Can you work these out from the model? Positions are in its coordinate system, mm. A direction names the side the tool comes from. Round coordinates to 2 decimals unless told otherwise and drop trailing zeros. Write each loop counter-clockwise with the first axis right and the second up, starting at its lowest first coordinate (ties: lowest second). Pieces come first, ordered by that corner, then holes. Notation, with made-up numbers: M 26,-21 L 35,-21 A11 ccw 35,-17 Z; hole C 66.5,-24 d3. An arc over 180 degrees is marked long. Answer as a JSON object with one key per item and string values. Group by question number.
1) Please list where these lines run through material, in increasing order: L1, parallel to Y at x = 15.5, z = 42.75; L2, parallel to X at y = -15, z = 44. Write a range as [from, to].
2) On a 3-axis mill with a long thin cutter (end or side, diameter ignored), from which of +Z, -Z, +X, -X, +Y, -Y can I reach the whole of each face in a straight line? I mean faces 4 (the cylindrical face through (16.421, 16.345, 43.237)), 5 (the flat face through (8, 23, 4)), 6 (the flat face through (0, -20, 24)). Say none if no direction works.
3) If we mould it in two halves opening along Z, with no side actions, what happens to faces 1 (the conical face through (-15.55, 15.29, 38.18)), 2 (the flat face through (0, -21, 5)), 3 (the flat face through (20.3, 0.1, 10))? For each: +Z half, -Z half, draft (parallel to the pull), parting line (faces both ways), or undercut.
4) I'm going to push flat-ended pins straight in: pin 1 Ø11 at (x, z) = (-0.5, 42.5) entering from +Y; pin 2 Ø10 at (x, y) = (9, 1) entering from +Z; pin 3 Ø1.5 at (x, y) = (-1, -15.5) entering from +Z. Where does each tip first touch, or does it pass through?
5) Suppose I cut it at A-A, the plane z = 46. Write out the boundary of the cut face in (x, y).
6) Suppose I cut it at B-B, the plane y = 0. Write out the boundary of the cut face in (x, z).
from build123d import *

# Parameters (mm, degrees)
EXTRUDE_1_DEPTH        = 10
EXTRUDE_2_DEPTH        = 27.8
EXTRUDE_3_DEPTH        = 10
SKETCH_4_R             = 11
EXTRUDE_4_DEPTH        = 2
SKETCH_5_R             = 2.5
EXTRUDE_5_DEPTH        = 18
FILLET_1_R             = 0.5
FILLET_2_R             = 0.8
FILLET_3_R             = 1
FILLET_4_R             = 1
HOLE_WIZARD_M3_4_D     = 2.5
HOLE_WIZARD_M3_4_DEPTH = 9
HOLE_WIZARD_M3_4_TIP   = 0.751075774
SKETCH_18_W            = 16
SKETCH_18_H            = 4
EXTRUDE_6_DEPTH        = 4
SKETCH_19_W            = 16
SKETCH_19_H            = 5
EXTRUDE_7_DEPTH        = 5
SKETCH_20_W            = 15
SKETCH_20_H            = 4
CUT_EXTRUDE_2_DEPTH    = 4.5
SKETCH_22_W            = 9
SKETCH_22_H            = 4.5
CUT_EXTRUDE_3_DEPTH    = 0.5
SKETCH_23_W            = 0.5
SKETCH_23_H            = 0.5
EXTRUDE_8_DEPTH        = 4.5
FILLET_6_R             = 0.1
FILLET_7_R             = 0.1
FILLET_8_R             = 0.1
FILLET_9_R             = 0.1
FILLET_10_R            = 0.1
FILLET_11_R            = 0.1


with BuildPart() as part:
    # 草图1 → 凸台-拉伸1 (new body)
    with BuildSketch(Plane.XY):
        Polygon((15.5, 21), (21, 15.5), (21, -15.5), (15.5, -21), (-15.5, -21), (-21, -15.5), (-21, 15.5), (-15.5, 21), align=None)
    extrude(amount=EXTRUDE_1_DEPTH)

    # 草图2 → 凸台-拉伸2 (add)
    with BuildSketch(Plane.XY.offset(10)):
        with BuildLine():
            Line((-11, 20), (11, 20))
            add(Edge.make_bspline(
                [(11, 20), (13.640929295, 20), (17.12066085, 17.472562842), (20, 12.937125311), (20, 11)],
                knots=[0, 0, 0, 0, 0.5, 1, 1, 1, 1], degree=3))
            Line((20, 11), (20, -11))
            add(Edge.make_bspline(
                [(20, -11), (20, -13.640929295), (17.472562842, -17.12066085), (12.937125311, -20), (11, -20)],
                knots=[0, 0, 0, 0, 0.5, 1, 1, 1, 1], degree=3))
            Line((11, -20), (-11, -20))
            add(Edge.make_bspline(
                [(-11, -20), (-13.640929295, -20), (-17.12066085, -17.472562842), (-20, -12.937125311), (-20, -11)],
                knots=[0, 0, 0, 0, 0.5, 1, 1, 1, 1], degree=3))
            Line((-20, -11), (-20, 11))
            add(Edge.make_bspline(
                [(-20, 11), (-20, 13.640929295), (-17.472562842, 17.12066085), (-12.937125311, 20), (-11, 20)],
                knots=[0, 0, 0, 0, 0.5, 1, 1, 1, 1], degree=3))
        make_face()
    extrude(amount=EXTRUDE_2_DEPTH)

    # 草图3 → 凸台-拉伸3 (add)
    with BuildSketch(Plane.XY.offset(37.8)):
        Polygon((21, -15.5), (21, 15.5), (15.5, 21), (-15.5, 21), (-21, 15.5), (-21, -15.5), (-15.5, -21), (15.5, -21), align=None)
    extrude(amount=EXTRUDE_3_DEPTH)

    # 草图4 → 凸台-拉伸4 (add)
    with BuildSketch(Plane.XY.offset(47.8)):
        Circle(SKETCH_4_R)
    extrude(amount=EXTRUDE_4_DEPTH)

    # 草图5 → 凸台-拉伸5 (add)
    with BuildSketch(Plane.XY.offset(49.8)):
        Circle(SKETCH_5_R)
    extrude(amount=EXTRUDE_5_DEPTH)

    # 圆角1
    fillet_1_edges = [part.edges().sort_by_distance(p)[0] for p in [
        (-2.5, 0, 67.8),
    ]]
    fillet(fillet_1_edges, radius=FILLET_1_R)

    # 圆角2
    fillet_2_edges = [part.edges().sort_by_distance(p)[0] for p in [
        (-11, 0, 49.8),
    ]]
    fillet(fillet_2_edges, radius=FILLET_2_R)

    # 圆角3
    fillet_3_edges = [part.edges().sort_by_distance(p)[0] for p in [
        (21, -15.5, 5),
        (15.5, -21, 5),
        (-15.5, -21, 5),
        (-21, -15.5, 5),
        (-21, 15.5, 5),
        (-15.5, 21, 5),
        (15.5, 21, 5),
        (21, 15.5, 5),
    ]]
    fillet(fillet_3_edges, radius=FILLET_3_R)

    # 圆角4
    fillet_4_edges = [part.edges().sort_by_distance(p)[0] for p in [
        (21, 15.5, 42.8),
        (15.5, 21, 42.8),
        (-15.5, 21, 42.8),
        (-21, 15.5, 42.8),
        (-21, -15.5, 42.8),
        (-15.5, -21, 42.8),
        (15.5, -21, 42.8),
        (21, -15.5, 42.8),
    ]]
    fillet(fillet_4_edges, radius=FILLET_4_R)

    # M3 螺纹孔4
    with Locations(Plane(origin=(-15.5, 15.5, 47.8), x_dir=(1, 0, 0), z_dir=(0, 0, 1))):
        with Locations((0, 0), (31, 0), (31, -31), (0, -31)):
            Hole(HOLE_WIZARD_M3_4_D / 2, depth=HOLE_WIZARD_M3_4_DEPTH)
            with Locations((0, 0, -(HOLE_WIZARD_M3_4_DEPTH + HOLE_WIZARD_M3_4_TIP / 2))):  # 118° drill point
                Cone(0, HOLE_WIZARD_M3_4_D / 2, HOLE_WIZARD_M3_4_TIP, mode=Mode.SUBTRACT)

    # 草图18 → 凸台-拉伸6 (add)
    with BuildSketch(Plane(origin=(0, 0, 0), x_dir=(-1, 0, 0), z_dir=(0, 0, -1))):
        with Locations((0, 23)):
            Rectangle(SKETCH_18_W, SKETCH_18_H)
    extrude(amount=-EXTRUDE_6_DEPTH)

    # 草图19 → 凸台-拉伸7 (add)
    with BuildSketch(Plane.XY.offset(4)):
        with Locations((0, 23.5)):
            Rectangle(SKETCH_19_W, SKETCH_19_H)
    extrude(amount=EXTRUDE_7_DEPTH)

    # 草图20 → 切除-拉伸2 (cut)
    with BuildSketch(Plane(origin=(0, 26, 0), x_dir=(1, 0, 0), z_dir=(0, 1, 0))):
        with Locations((0, -6.5)):
            Rectangle(SKETCH_20_W, SKETCH_20_H)
    extrude(amount=-CUT_EXTRUDE_2_DEPTH, mode=Mode.SUBTRACT)

    # 草图22 → 切除-拉伸3 (cut)
    with BuildSketch(Plane.XY.offset(9)):
        with Locations((0, 23.75)):
            Rectangle(SKETCH_22_W, SKETCH_22_H)
    extrude(amount=-CUT_EXTRUDE_3_DEPTH, mode=Mode.SUBTRACT)

    # 草图23 → 凸台-拉伸8 (add)
    with BuildSketch(Plane(origin=(0, 21.5, 0), x_dir=(1, 0, 0), z_dir=(0, 1, 0))):
        with Locations((-3.21, -6.5)):
            Rectangle(SKETCH_23_W, SKETCH_23_H)
        with Locations((-5.35, -6.5)):
            Rectangle(SKETCH_23_W, SKETCH_23_H)
        with Locations((-1.07, -6.5)):
            Rectangle(SKETCH_23_W, SKETCH_23_H)
        with Locations((1.07, -6.5)):
            Rectangle(SKETCH_23_W, SKETCH_23_H)
        with Locations((3.21, -6.5)):
            Rectangle(SKETCH_23_W, SKETCH_23_H)
        with Locations((5.35, -6.5)):
            Rectangle(SKETCH_23_W, SKETCH_23_H)
    extrude(amount=EXTRUDE_8_DEPTH)

    # 圆角6
    fillet_6_edges = [part.edges().sort_by_distance(p)[0] for p in [
        (-5.6, 23.75, 6.75),
        (-5.6, 23.75, 6.25),
        (-5.1, 23.75, 6.25),
        (-5.1, 23.75, 6.75),
    ]]
    fillet(fillet_6_edges, radius=FILLET_6_R)

    # 圆角7
    fillet_7_edges = [part.edges().sort_by_distance(p)[0] for p in [
        (-3.46, 23.75, 6.25),
        (-2.96, 23.75, 6.25),
        (-2.96, 23.75, 6.75),
        (-3.46, 23.75, 6.75),
    ]]
    fillet(fillet_7_edges, radius=FILLET_7_R)

    # 圆角8
    fillet_8_edges = [part.edges().sort_by_distance(p)[0] for p in [
        (-1.32, 23.75, 6.25),
        (-0.82, 23.75, 6.25),
        (-0.82, 23.75, 6.75),
        (-1.32, 23.75, 6.75),
    ]]
    fillet(fillet_8_edges, radius=FILLET_8_R)

    # 圆角9
    fillet_9_edges = [part.edges().sort_by_distance(p)[0] for p in [
        (0.82, 23.75, 6.25),
        (1.32, 23.75, 6.25),
        (1.32, 23.75, 6.75),
        (0.82, 23.75, 6.75),
    ]]
    fillet(fillet_9_edges, radius=FILLET_9_R)

    # 圆角10
    fillet_10_edges = [part.edges().sort_by_distance(p)[0] for p in [
        (2.96, 23.75, 6.25),
        (3.46, 23.75, 6.25),
        (3.46, 23.75, 6.75),
        (2.96, 23.75, 6.75),
    ]]
    fillet(fillet_10_edges, radius=FILLET_10_R)

    # 圆角11
    fillet_11_edges = [part.edges().sort_by_distance(p)[0] for p in [
        (5.1, 23.75, 6.25),
        (5.6, 23.75, 6.25),
        (5.6, 23.75, 6.75),
        (5.1, 23.75, 6.75),
    ]]
    fillet(fillet_11_edges, radius=FILLET_11_R)


solid = part.part
Results:
{
 "1": {"L1": "[-20.91, -16.75], [-14.25, 14.25], [16.75, 20.91]", "L2": "[-21, -16.65], [-14.35, 14.35], [16.65, 21]"},
 "2": {"face 4": "+Z", "face 5": "+Z, -Z, +X, +Y", "face 6": "+X, -X, -Y"},
 "3": {"face 1": "+Z half", "face 2": "draft", "face 3": "undercut"},
 "4": {"pin 1": "y = 21", "pin 2": "z = 49.8", "pin 3": "z = 47.8"},
 "5": {"outline": "M -21,-15.09 A1 ccw -20.71,-15.79 L -15.79,-20.71 A1 ccw -15.09,-21 L 15.09,-21 A1 ccw 15.79,-20.71 L 20.71,-15.79 A1 ccw 21,-15.09 L 21,15.09 A1 ccw 20.71,15.79 L 15.79,20.71 A1 ccw 15.09,21 L -15.09,21 A1 ccw -15.79,20.71 L -20.71,15.79 A1 ccw -21,15.09 Z; hole C -15.5,-15.5 d2.5; hole C -15.5,15.5 d2.5; hole C 15.5,-15.5 d2.5; hole C 15.5,15.5 d2.5"},
 "6": {"outline": "M -21,0 L 21,0 L 21,10 L 20,10 L 20,37.8 L 21,37.8 L 21,47.8 L 11,47.8 L 11,49 A0.8 ccw 10.2,49.8 L 2.5,49.8 L 2.5,67.3 A0.5 ccw 2,67.8 L -2,67.8 A0.5 ccw -2.5,67.3 L -2.5,49.8 L -10.2,49.8 A0.8 ccw -11,49 L -11,47.8 L -21,47.8 L -21,37.8 L -20,37.8 L -20,10 L -21,10 Z"}
}
